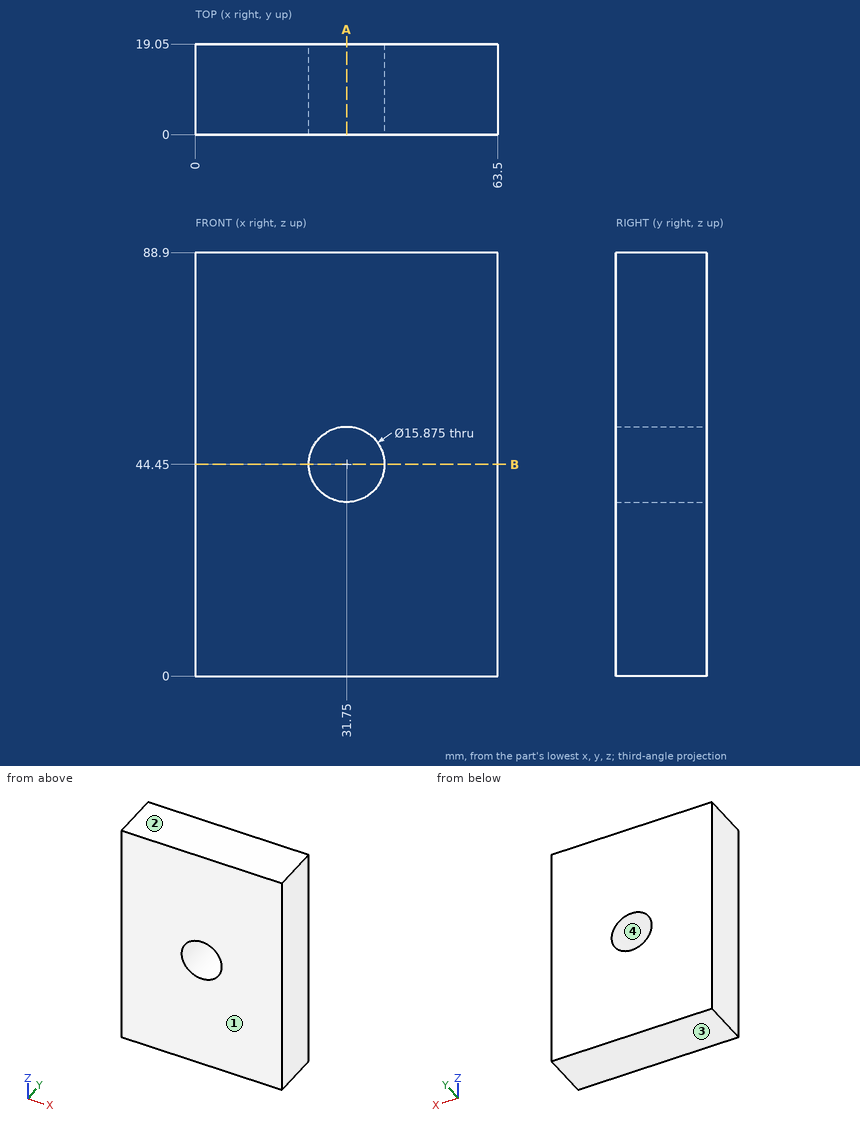
Print and shaded views of the part. All mm, measured from the part's lowest x, y and z. Coordinates: 2 decimals unless noted, no trailing zeros. Loops run counter-clockwise (first coordinate to the right, second up) from the corner with the lowest first, then second, coordinate; pieces in that order, holes last. Notation, with made-up numbers: (1, 74.25) - (47, 74.25) arc R32 cw to (47, 105.25) - close; hole circle Ø5 at (-10, 87). An arc over 180 degrees is marked (long way). Write item = value, one per line. Start each with the question number.
Item 1: Saw through at B-B, the plane z = 44.45. List the corners of the cut face in (x, y), then the cut area to 3 significant figures.
Item 2: Pull direction Z, two halves, no side cores. Call the marked faces 1, 2, 3 and 4: +Z half, -Z half, draft (parallel to the pull), parting line (faces both ways), or undercut.
Item 3: Saw through at A-A, the plane x = 31.75. List the corners of the cut face in (y, z), then the cut area to 3 significant figures.
Item 4: Wall check: probe 1 along X at (y, z) = (14.5, 44.45); probe 2 along Z at (x, y) = (31.75, 15); probe 3 along Z at (x, y) = (25.5, 8). Give the ranges that are in metal, low to high. Write a range as [from, to].
Answers:
q1.outline = (0, 0) - (23.81, 0) - (23.81, 19.05) - (0, 19.05) - close; (39.69, 0) - (63.5, 0) - (63.5, 19.05) - (39.69, 19.05) - close
q1.area = 907 mm2
q2.face_1 = draft
q2.face_2 = +Z half
q2.face_3 = -Z half
q2.face_4 = undercut
q3.outline = (0, 0) - (19.05, 0) - (19.05, 36.51) - (0, 36.51) - close; (0, 52.39) - (19.05, 52.39) - (19.05, 88.9) - (0, 88.9) - close
q3.area = 1,390 mm2
q4.probe_1 = [0, 23.81], [39.69, 63.5]
q4.probe_2 = [0, 36.51], [52.39, 88.9]
q4.probe_3 = [0, 39.56], [49.34, 88.9]
